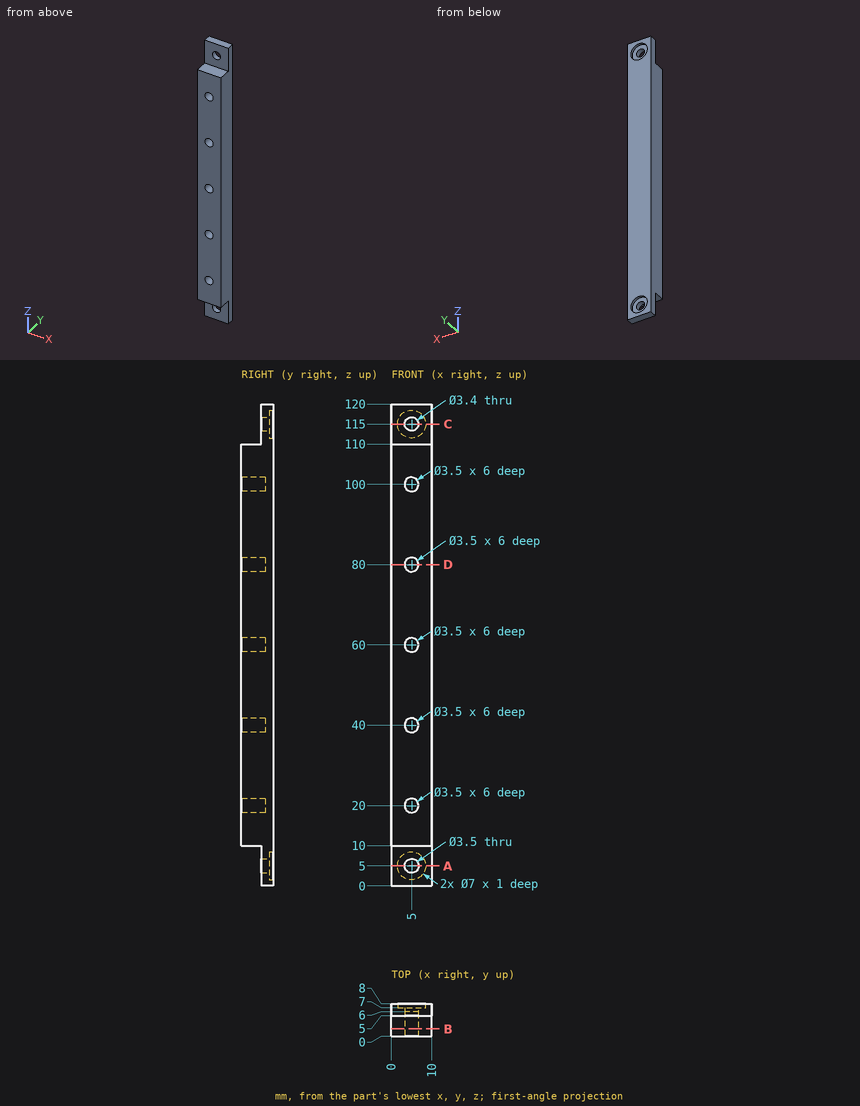
Geometry: see drawing. Coordinates: mm, zero at the bounding-box minimum. Give positions to 0.01 mm unless a question says otherwise; leave off trailing zeros. Order: outer loops, then holes, each group sorted by start corner. A loop starts at its lowest first (then second) coordinate and runs counter-clockwise, first axis right, second up. Notation, with made-up numbers: (-3.75, 8) -> (43.25, 8) arc R27 cw to (43.25, 43) -> close; hole circle Ø9 at (24.5, 67). An arc over 180 degrees is marked (long way). Write each question's results on one line, items separated by ' | '. Start each with the question number.
1) Section D-D (z = 80). Return loops of the section in (x, y), then the cut area to 3 significant figures.
2) Line query: line 1 (Z direction, x = 5, y = 4.65); line 2 (Z direction, x = 5, y = 7.45); line 3 (X direction, y = 3.75, z = 80). Output: solid intervals per line, ascending. Write a range as from..to.
3) Section B-B (y = 1.75). Return loops of the section in (x, z), then the cut area to 3 significant figures.
4) Section C-C (z = 115). Return loops of the section in (x, y), then the cut area to 3 significant figures.
5) Section A-A (z = 5). Return loops of the section in (x, y), then the cut area to 3 significant figures.
6) First-contact query: pin 1 (5.5 mm diameter, centred on x = 5, z = 5, fed in from -Y); pin 2 (1.5 mm diameter, centred on x = 4.5, y = 2.5, fed in from +Z); pin 3 (4.5 mm diameter, centred on x = 5, z = 40, fed in from -Y); pin 4 (1.8 mm diameter, centred on x = 5, z = 40.5, fed in from -Y). Flat tips, straight axial feed; report the tip coordinate or a pass-through.
Calculated:
1) outline: (0, 0) -> (3.25, 0) -> (3.25, 6) -> (6.75, 6) -> (6.75, 0) -> (10, 0) -> (10, 8) -> (0, 8) -> close | area: 59.0 mm2
2) line 1: 10..18.25, 21.75..38.25, 41.75..58.25, 61.75..78.25, 81.75..98.25, 101.75..110 | line 2: 0..1.5, 8.5..111.5, 118.5..120 | line 3: 0..3.25, 6.75..10
3) outline: (0, 10) -> (10, 10) -> (10, 110) -> (0, 110) -> close; hole circle Ø3.5 at (5, 20); hole circle Ø3.5 at (5, 40); hole circle Ø3.5 at (5, 60); hole circle Ø3.5 at (5, 80); hole circle Ø3.5 at (5, 100) | area: 952 mm2
4) outline: (0, 5) -> (3.3, 5) -> (3.3, 7) -> (1.5, 7) -> (1.5, 8) -> (0, 8) -> close; (6.7, 5) -> (10, 5) -> (10, 8) -> (8.5, 8) -> (8.5, 7) -> (6.7, 7) -> close | area: 16.2 mm2
5) outline: (0, 5) -> (3.25, 5) -> (3.25, 7) -> (1.5, 7) -> (1.5, 8) -> (0, 8) -> close; (6.75, 5) -> (10, 5) -> (10, 8) -> (8.5, 8) -> (8.5, 7) -> (6.75, 7) -> close | area: 16.0 mm2
6) pin 1: y = 5 | pin 2: z = 110 | pin 3: y = 0 | pin 4: y = 6
